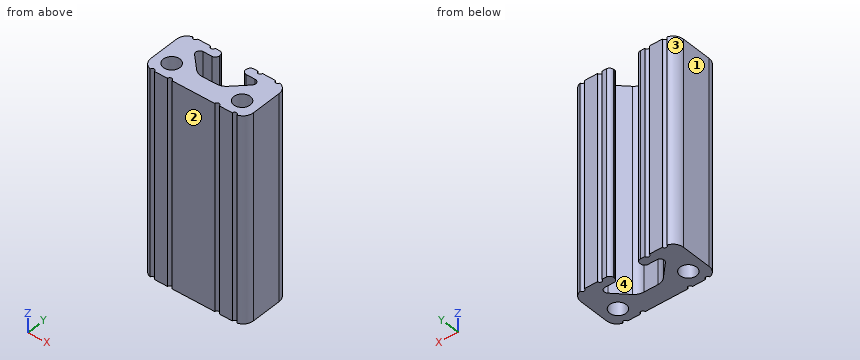
from build123d import *

# Parameters (mm, degrees)
SKETCH3_R               = 2.032
BOSS_EXTRUDE1_DEPTH     = 152.4
CUT_EXTRUDE1_DEPTH      = 154.060029074
CUT_EXTRUDE1_DEPTH_BACK = 154.060029074
SKETCH4_R               = 0.55245
CUT_EXTRUDE2_DEPTH      = 254


with BuildPart() as part:
    # Sketch3 → Boss-Extrude1 (new, symmetric)
    with BuildSketch(Plane.XY):
        with BuildLine():
            Line((3.2512, 5.35559), (3.2512, 5.13461))
            ThreePointArc((3.2512, 5.13461), (3.542455946, 4.431455946), (4.24561, 4.1402))
            Line((4.24561, 4.1402), (6.42239, 4.1402))
            ThreePointArc((6.42239, 4.1402), (7.341105046, 3.526334232), (7.125544054, 2.442635946))
            Line((7.125544054, 2.442635946), (3.854875946, -0.828032163))
            ThreePointArc((3.854875946, -0.828032163), (2.887046479, -1.474715138), (1.745413783, -1.7018))
            Line((1.745413783, -1.7018), (0, -1.7018))
            Line((0, -1.7018), (0, -6.35))
            Line((0, -6.35), (10.16, -6.35))
            ThreePointArc((10.16, -6.35), (11.956051224, -5.606051224), (12.7, -3.81))
            Line((12.7, -3.81), (12.7, 3.81))
            ThreePointArc((12.7, 3.81), (11.956051224, 5.606051224), (10.16, 6.35))
            Line((10.16, 6.35), (4.24561, 6.35))
            ThreePointArc((4.24561, 6.35), (3.542455946, 6.058744054), (3.2512, 5.35559))
        make_face()
        with Locations(Location((8.7249, -2.3876, 0), (0, 0, 180))):
            Circle(SKETCH3_R, mode=Mode.SUBTRACT)
    extrude(amount=BOSS_EXTRUDE1_DEPTH, both=True)

    # Sketch4 → Cut-Extrude1 (cut, two sides: drawn at the far end of the back side and taken through both)
    with BuildSketch(Plane.XY.offset(-CUT_EXTRUDE1_DEPTH_BACK)):
        with Locations((5.86994, 6.35)):
            Circle(SKETCH4_R)
        with Locations((10.20445, 6.35)):
            Circle(SKETCH4_R)
        with Locations((5.86994, -6.35)):
            Circle(SKETCH4_R)
        with Locations((10.20445, -6.35)):
            Circle(SKETCH4_R)
    extrude(amount=CUT_EXTRUDE1_DEPTH + CUT_EXTRUDE1_DEPTH_BACK, mode=Mode.SUBTRACT)

    # Mirror1: part across plane


with BuildPart() as part_1:
    add(part.part)
    add(part.part.mirror(Plane(origin=(0, 0, 0), x_dir=(0, 0, 1), z_dir=(1, 0, 0))))

    # Sketch5 → Cut-Extrude2 (cut)
    with BuildSketch(Plane.XY.offset(152.4)):
        with BuildLine():
            Line((9.652, 6.35), (6.42239, 6.35))
            ThreePointArc((6.42239, 6.35), (5.86994, 5.79755), (5.31749, 6.35))
            Line((5.31749, 6.35), (4.24561, 6.35))
            ThreePointArc((4.24561, 6.35), (3.542455946, 6.058744054), (3.2512, 5.35559))
            Line((3.2512, 5.35559), (3.2512, 5.13461))
            ThreePointArc((3.2512, 5.13461), (3.542455946, 4.431455946), (4.24561, 4.1402))
            Line((4.24561, 4.1402), (6.42239, 4.1402))
            ThreePointArc((6.42239, 4.1402), (7.341105046, 3.526334232), (7.125544054, 2.442635946))
            Line((7.125544054, 2.442635946), (3.854875946, -0.828032163))
            ThreePointArc((3.854875946, -0.828032163), (2.887046479, -1.474715138), (1.745413783, -1.7018))
            Line((1.745413783, -1.7018), (-1.745413783, -1.7018))
            ThreePointArc((-1.745413783, -1.7018), (-2.887046479, -1.474715138), (-3.854875946, -0.828032163))
            Line((-3.854875946, -0.828032163), (-7.125544054, 2.442635946))
            ThreePointArc((-7.125544054, 2.442635946), (-7.341105046, 3.526334232), (-6.42239, 4.1402))
            Line((-6.42239, 4.1402), (-4.24561, 4.1402))
            ThreePointArc((-4.24561, 4.1402), (-3.542455946, 4.431455946), (-3.2512, 5.13461))
            Line((-3.2512, 5.13461), (-3.2512, 5.35559))
            ThreePointArc((-3.2512, 5.35559), (-3.542455946, 6.058744054), (-4.24561, 6.35))
            Line((-4.24561, 6.35), (-5.31749, 6.35))
            ThreePointArc((-5.31749, 6.35), (-5.86994, 5.79755), (-6.42239, 6.35))
            Line((-6.42239, 6.35), (-9.652, 6.35))
            ThreePointArc((-9.652, 6.35), (-10.169350236, 5.798666155), (-10.752439892, 6.279942302))
            ThreePointArc((-10.752439892, 6.279942302), (-12.154542219, 5.382705102), (-12.7, 3.81))
            Line((-12.7, 3.81), (-12.7, -3.81))
            ThreePointArc((-12.7, -3.81), (-12.154542219, -5.382705102), (-10.752439892, -6.279942302))
            ThreePointArc((-10.752439892, -6.279942302), (-10.169350236, -5.798666155), (-9.652, -6.35))
            Line((-9.652, -6.35), (-6.42239, -6.35))
            ThreePointArc((-6.42239, -6.35), (-5.86994, -5.79755), (-5.31749, -6.35))
            Line((-5.31749, -6.35), (5.31749, -6.35))
            ThreePointArc((5.31749, -6.35), (5.86994, -5.79755), (6.42239, -6.35))
            Line((6.42239, -6.35), (9.652, -6.35))
            ThreePointArc((9.652, -6.35), (10.169350236, -5.798666155), (10.752439892, -6.279942302))
            ThreePointArc((10.752439892, -6.279942302), (12.154542219, -5.382705102), (12.7, -3.81))
            Line((12.7, -3.81), (12.7, 3.81))
            ThreePointArc((12.7, 3.81), (12.154542219, 5.382705102), (10.752439892, 6.279942302))
            ThreePointArc((10.752439892, 6.279942302), (10.169350236, 5.798666155), (9.652, 6.35))
        make_face()
    extrude(amount=-CUT_EXTRUDE2_DEPTH, mode=Mode.SUBTRACT)


solid = part_1.part
For this review, take the finished solid that the model builds, in its own axes (mm). Face numbers are marked on the shaded views. Round coordinates to 2 decimals unless told otherwise and drop trailing zeros. Loops run counter-clockwise (first coordinate to the right, second up) from the corner with the lowest first, then second, coordinate; pieces in that order, holes last. Notation, with made-up numbers: (0.25, 80.25) - (19.25, 80.25) arc R29 ccw to (19.25, 109.25) - close; hole circle Ø1 at (5, -35). An arc over 180 degrees is marked (long way). Put each result on its own line as item: value. Start each with the question number.
1. Consider section D-D on x = -0.25. State the section outline as (y, z) points.
2. Consider section A-A on x = -8.5. State the section outline as (y, z) points, plus the area to 3 significant figures.
3. For probe 1 along Y at (x, z) = (8.5, -120); probe 2 along X at (y, z) = (-2, -131); probe 3 along Y at (x, z) = (7, -145.5), list the stretches that pass through material, from the lowest coordinate up. Write a range as [from, to].
4. Consider section B-B on y = 0.75. State the section outline as (x, z) points.
5. Consider section C-C on y = -3.25. State the section outline as (x, z) points.
6. Insertion check: P1, Ø5, axis at x = 0.5, z = -114.5, coming from the +Y side; P2, Ø1.7, axis at x = 0.5, z = -131.5, coming from the +Y side. Each pin has a flat end and moves straight along its axis. Give the tip position at first contact, or say it passes through.
7. Mouldability with a two-part tool opening along Y and no side actions: class the marked faces 1, 2, 3 and 4 as +Y half, -Y half, draft (parallel to the pull), parting line (faces both ways), or undercut.
Result sheet:
1. outline: (-6.35, -152.4) - (-1.7, -152.4) - (-1.7, -101.6) - (-6.35, -101.6) - close
2. outline: (-6.35, -152.4) - (-4.41, -152.4) - (-4.41, -101.6) - (-6.35, -101.6) - close; (-0.37, -152.4) - (6.35, -152.4) - (6.35, -101.6) - (-0.37, -101.6) - close
2. area: 440 mm^2
3. probe 1: [-6.35, -4.41], [-0.37, 6.35]
3. probe 2: [-12.7, -10.72], [-6.73, 6.73], [10.72, 12.7]
3. probe 3: [-6.35, -3.46], [-1.31, 2.32], [3.96, 6.35]
4. outline: (-12.7, -152.4) - (-5.43, -152.4) - (-5.43, -101.6) - (-12.7, -101.6) - close; (5.43, -152.4) - (12.7, -152.4) - (12.7, -101.6) - (5.43, -101.6) - close
5. outline: (-12.7, -152.4) - (-10.56, -152.4) - (-10.56, -101.6) - (-12.7, -101.6) - close; (-6.88, -152.4) - (6.88, -152.4) - (6.88, -101.6) - (-6.88, -101.6) - close; (10.56, -152.4) - (12.7, -152.4) - (12.7, -101.6) - (10.56, -101.6) - close
6. P1: y = -1.43
6. P2: y = -1.7
7. face 1: draft
7. face 2: -Y half
7. face 3: +Y half
7. face 4: undercut
